Check sheet for the drawn part. Datum: minimum x, y, z corner. Units: mm. A direction names the side the tool comes from. Coordinates: 2 decimals unless noted, no trailing zeros. Order: outer loops, then holes, each group sorted by start corner. A loop starts at its lowest first (then second) coordinate and runs counter-clockwise, first axis right, second up.
Q1. Cross-section at B-B, the plane z = 40. Record the boundary of the cut face in (x, y), and give its area (3 significant figures).
Q2. Depth check by flat-ended pin: P1, Ø3, axis at y = 63.5, z = 75, coming from the +X side; P2, Ø8, axis at y = 108.5, z = 53, coming from the +X side; P3, Ø12, axis at y = 126, z = 25.5, coming from the -X side; P4, Ø1, axis at x = 68.5, y = 105, coming from the +Z side. Enter the tip coordinate at first touch or a pass-through.
Q3. Cross-section at D-D, the plane y = 115.5. Record the boundary of the cut face in (x, z).
Q4. Thickness scan on line 1 (Y direction, x = 45, z = 87); line 2 (Z direction, x = 31, y = 42.5) (1 decimal); line 3 (X direction, y = 111, z = 12) (1 decimal). Record the ranges inside material, lowest first.
Q5. Set-up check for the marked faces 1 and 2: record each of +Z, -Z, +X, -X, +Y, -Y from which the full face is reachable in a straight line by a thin tool's end or side.
Q6. Cross-section at A-A, the plane x = 84.5. Record the boundary of the cut face in (y, z), and give its area (3 significant figures).
Q7. Cross-section at C-C, the plane y = 46. Record the boundary of the cut face in (x, z) (1 decimal), and give its area (3 significant figures).
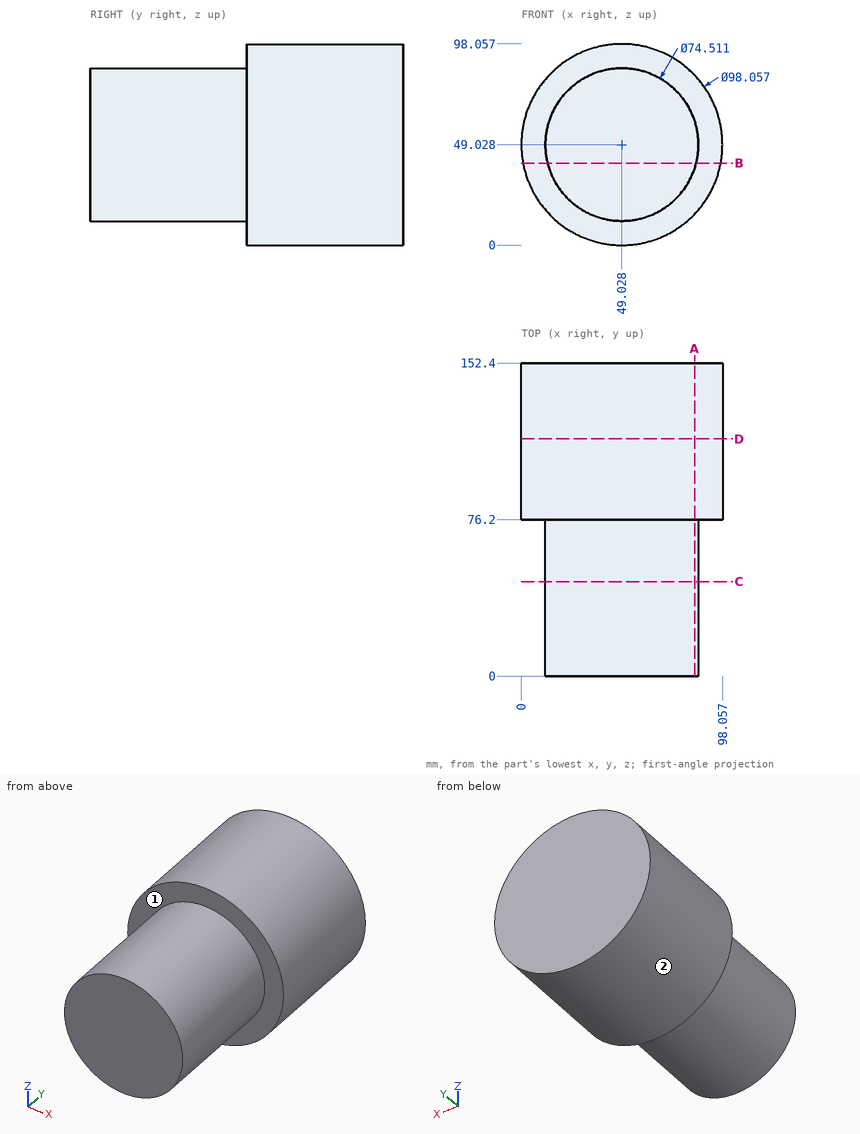
Check values:
1. outline: (0.84, 76.2) - (12.88, 76.2) - (12.88, 0) - (85.17, 0) - (85.17, 76.2) - (97.22, 76.2) - (97.22, 152.4) - (0.84, 152.4) - close
1. area: 12,900 mm2
2. P1: stops at x = 77.12
2. P2: stops at x = 98.06
2. P3: stops at x = 3.24
2. P4: stops at z = 94.24
3. outline: circle Ø98.06 at (49.03, 49.03)
4. line 1: y = 76.2 to 152.4
4. line 2: z = 16.4 to 81.6
4. line 3: x = 16.9 to 81.2
5. face 1: -Y
5. face 2: +Y, -Y
6. outline: (0, 37.64) - (76.2, 37.64) - (76.2, 15.18) - (152.4, 15.18) - (152.4, 82.87) - (76.2, 82.87) - (76.2, 60.42) - (0, 60.42) - close
6. area: 6,890 mm2
7. outline: circle Ø74.5 at (49, 49)
7. area: 4,360 mm2
